Geometry check sheet. Reference: the model listing, model coordinates, mm. Coordinates: 2 decimals unless noted, no trailing zeros. Write each loop counter-clockwise with the first axis right and the second up, starting at its lowest first coordinate (ties: lowest second). Pieces come first, ordered by that corner, then holes. Notation, with made-up numbers: M -11.75,-16 L 5.25,-16 A15 ccw 5.25,3 Z; hole C 88.5,-38.75 d4. An arc over 180 degrees is marked long. Write item = value, one per line. Start each with the question number.
```python
from build123d import *

# Parameters (mm, degrees)
SKETCH1_R           = 1.55
BOSS_EXTRUDE1_DEPTH = 1.5
FILLET1_R           = 6
SKETCH2_W           = 4
SKETCH2_H           = 5
BOSS_EXTRUDE2_DEPTH = 1
SKETCH3_W           = 1.405588528
SKETCH3_H           = 1.405588528
BOSS_EXTRUDE3_DEPTH = 0.5


with BuildPart() as part:
    # Sketch1 → Boss-Extrude1 (new body)
    with BuildSketch(Plane(origin=(0, 0, 0), x_dir=(1, 0, 0), z_dir=(0, 1, 0))):
        with BuildLine():
            Line((9.898679656, 14.141320344), (0, 4.242640687))
            Line((0, 4.242640687), (4.242640687, 0))
            Line((4.242640687, 0), (14.141320344, 9.898679656))
            ThreePointArc((14.141320344, 9.898679656), (14.141320344, 14.141320344), (9.898679656, 14.141320344))
        make_face()
        with Locations((12.02, 12.02)):
            Circle(SKETCH1_R, mode=Mode.SUBTRACT)
        with BuildLine():
            Line((-14.141320344, 9.898679656), (-4.242640687, 0))
            Line((-4.242640687, 0), (0, 4.242640687))
            Line((0, 4.242640687), (-9.898679656, 14.141320344))
            ThreePointArc((-9.898679656, 14.141320344), (-14.141320344, 14.141320344), (-14.141320344, 9.898679656))
        make_face()
        with Locations((-12.02, 12.02)):
            Circle(SKETCH1_R, mode=Mode.SUBTRACT)
        Polygon((0, 4.242640687), (-4.242640687, 0), (0, -4.242640687), (4.242640687, 0), align=None)
        with BuildLine():
            Line((4.242640687, 0), (0, -4.242640687))
            Line((0, -4.242640687), (9.898679656, -14.141320344))
            ThreePointArc((9.898679656, -14.141320344), (14.141320344, -14.141320344), (14.141320344, -9.898679656))
            Line((14.141320344, -9.898679656), (4.242640687, 0))
        make_face()
        with Locations((12.02, -12.02)):
            Circle(SKETCH1_R, mode=Mode.SUBTRACT)
        with BuildLine():
            Line((-4.242640687, 0), (-14.141320344, -9.898679656))
            ThreePointArc((-14.141320344, -9.898679656), (-14.141320344, -14.141320344), (-9.898679656, -14.141320344))
            Line((-9.898679656, -14.141320344), (0, -4.242640687))
            Line((0, -4.242640687), (-4.242640687, 0))
        make_face()
        with Locations((-12.02, -12.02)):
            Circle(SKETCH1_R, mode=Mode.SUBTRACT)
    extrude(amount=BOSS_EXTRUDE1_DEPTH)

    # Fillet1
    fillet1_edges = [part.edges().sort_by_distance(p)[0] for p in [
        (4.242640687, 0.75, 0),
        (0, 0.75, 4.242640687),
        (-4.242640687, 0.75, 0),
        (0, 0.75, -4.242640687),
    ]]
    fillet(fillet1_edges, radius=FILLET1_R)

    # Sketch2 → Boss-Extrude2 (add)
    with BuildSketch(Plane(origin=(0, 1.5, 0), x_dir=(1, 0, 0), z_dir=(0, 1, 0))):
        Rectangle(SKETCH2_W, SKETCH2_H)
    extrude(amount=BOSS_EXTRUDE2_DEPTH)

    # Sketch3 → Boss-Extrude3 (add)
    with BuildSketch(Plane(origin=(0, 1.5, 0), x_dir=(1, 0, 0), z_dir=(0, 1, 0))):
        with Locations((-3.030370202, -1.797205736)):
            Rectangle(SKETCH3_W, SKETCH3_H)
        with Locations((-3.030370202, 0)):
            Rectangle(SKETCH3_W, SKETCH3_H)
        with Locations((-3.030370202, 1.797205736)):
            Rectangle(SKETCH3_W, SKETCH3_H)
        with Locations((3.108126605, 0)):
            Rectangle(SKETCH3_W, SKETCH3_H)
        with Locations((3.108126605, -1.797205736)):
            Rectangle(SKETCH3_W, SKETCH3_H)
        with Locations((3.108126605, 1.797205736)):
            Rectangle(SKETCH3_W, SKETCH3_H)
    extrude(amount=BOSS_EXTRUDE3_DEPTH)


solid = part.part
```
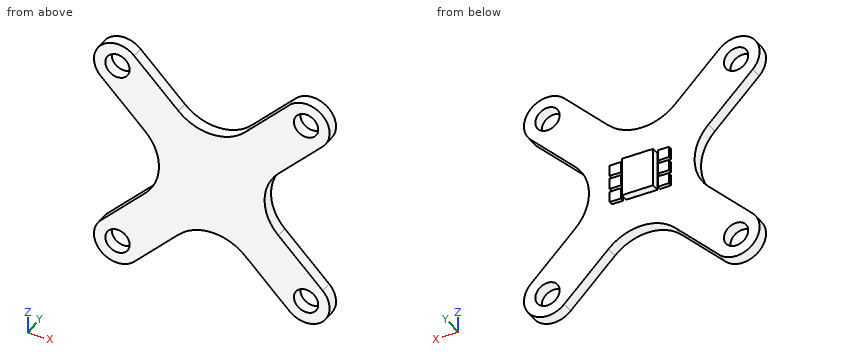
Q1. Cross-section at C-C on z = -12.02. Enter the section's corners in (x, y).
Q2. Scan lines: L1, parallel to X at y = 1.15, z = -12.02; L2, parallel to Z at x = 13, y = 0.5. Record each from-to range of solid material in increasing order.
Q3. Cross-section at D-D on x = 0.5. Enter the section's corners in (y, z), and give its area (3 significant figures).
Q4. Gauge pin test, flat ends, axial feed: pin 1 (4 mm diameter, centred on x = 12.02, z = -12.02, fed in from +Y); pin 2 (0.7 mm diameter, centred on x = -3, z = -2, fed in from +Y). Record the tip position at first contact, or that the pin passes through.
Q5. Cross-section at A-A on y = 0.6. Enter the section's corners in (x, z), and give its area (3 significant figures).
Q6. Cross-section at B-B on x = -12. Enter the section's corners in (y, z).
Values found:
q1.outline = M -15.02,0 L -13.57,0 L -13.57,1.5 L -15.02,1.5 Z; M -10.47,0 L -7.78,0 L -7.78,1.5 L -10.47,1.5 Z; M 7.78,0 L 10.47,0 L 10.47,1.5 L 7.78,1.5 Z; M 13.57,0 L 15.02,0 L 15.02,1.5 L 13.57,1.5 Z
q2.L1 = -15.02 to -13.57, -10.47 to -7.78, 7.78 to 10.47, 13.57 to 15.02
q2.L2 = -14.86 to -13.22, -10.82 to -8.76, 8.76 to 10.82, 13.22 to 14.86
q3.outline = M 0,-6.75 L 1.5,-6.75 L 1.5,-2.5 L 2.5,-2.5 L 2.5,2.5 L 1.5,2.5 L 1.5,6.75 L 0,6.75 Z
q3.area = 25.2 mm²
q4.pin_1 = 1.5
q4.pin_2 = 2
q5.outline = M -14.14,-9.9 A3 ccw -9.9,-14.14 L -4.24,-8.49 A6 cw 4.24,-8.49 L 9.9,-14.14 A3 ccw 14.14,-9.9 L 8.49,-4.24 A6 cw 8.49,4.24 L 14.14,9.9 A3 ccw 9.9,14.14 L 4.24,8.49 A6 cw -4.24,8.49 L -9.9,14.14 A3 ccw -14.14,9.9 L -8.49,4.24 A6 cw -8.49,-4.24 Z; hole C -12.02,-12.02 d3.1; hole C -12.02,12.02 d3.1; hole C 12.02,-12.02 d3.1; hole C 12.02,12.02 d3.1
q5.area = 429 mm²
q6.outline = M 0,-15.02 L 1.5,-15.02 L 1.5,-13.57 L 0,-13.57 Z; M 0,-10.47 L 1.5,-10.47 L 1.5,-7.76 L 0,-7.76 Z; M 0,7.76 L 1.5,7.76 L 1.5,10.47 L 0,10.47 Z; M 0,13.57 L 1.5,13.57 L 1.5,15.02 L 0,15.02 Z
